Autodesk Fusion 360 part; units mm, degrees
sketch "Sketch1" plane through (0, 0, 0) normal (0, 0, 1) x (1, 0, 0)
  line L0 (50.6391, 82.0886) -> (110.6391, 82.0886)
  line L1 (110.6391, 82.0886) -> (110.6391, 22.0886)
  line L2 (110.6391, 22.0886) -> (50.6391, 22.0886)
  line L3 (50.6391, 22.0886) -> (50.6391, 82.0886)
  line L4 (55.6391, 77.0886) -> (105.6391, 77.0886)
  line L5 (105.6391, 77.0886) -> (105.6391, 27.0886)
  line L6 (105.6391, 27.0886) -> (55.6391, 27.0886)
  line L7 (55.6391, 27.0886) -> (55.6391, 77.0886)
  dimension "d1" = 60
  dimension "d2" = 60
  dimension "d5" = 50
  dimension "d6" = 50
extrude "Extrude1" add sketch "Sketch1" along normal blind 10 contours L4 L5 L6 L7
extrude "Extrude2" add sketch "Sketch1" along normal blind 60
sketch "Sketch2" plane through (0, 22.0886, 0) normal (0, -1, 0) x (1, 0, 0)
  line L0 (50.6391, 0) -> (110.6391, 0)
  line L1 (110.6391, 0) -> (110.6391, 60)
  line L2 (110.6391, 60) -> (50.6391, 60)
  line L3 (50.6391, 60) -> (50.6391, 0)
  line L4 (80.6391, 35) -> (75.6391, 35)
  line L5 (75.6391, 35) -> (85.6391, 35)
  line L6 (85.6391, 35) -> (85.6391, 25)
  line L7 (85.6391, 25) -> (75.6391, 25)
  line L8 (75.6391, 25) -> (75.6391, 35)
  dimension "d13" = 10
  dimension "d14" = 10
extrude "Extrude3" cut sketch "Sketch2" against normal blind 3.3 contours L4 L5 L6 L7 L8
Input: part model. Units: mm. Frame: model coordinates. A direction names the side the tool comes from. Give positions to 0.01 mm unless a question says otherwise; leave off trailing zeros. Order: outer loops, then holes, each group sorted by start corner. A loop starts at its lowest first (then second) coordinate and runs counter-clockwise, first axis right, second up. Notation, with made-up numbers: (-9, 25.25) - (2, 25.25) arc R16 cw to (2, 48.25) - close; hole circle Ø10 at (-1, -29.5). An arc over 180 degrees is marked (long way). Use a Markdown table: item, result.
(1) Section query A-A (x = 104.5). Output: boundary loops of the cut face in (y, z), then the cut area to 3 significant figures.
Computed values:
| item | result |
|---|---|
| outline | (22.09, 0) - (82.09, 0) - (82.09, 60) - (77.09, 60) - (77.09, 10) - (27.09, 10) - (27.09, 60) - (22.09, 60) - close |
| area | 1,100 mm2 |
(2) Draft query along Z for faces 1 (the flat face through (80, 52, 10)), 2 (the flat face through (80, 53, 0)), 3 (the flat face through (81, 24, 25)), 4 (the flat face through (55.639, 52, 35)). Return one class per face: released by +Z, released by -Z, zero draft, split by the parting line, or undercut.
Computed values:
| item | result |
|---|---|
| face 1 | released by +Z |
| face 2 | released by -Z |
| face 3 | undercut |
| face 4 | zero draft |
(3) Pin query (flat end, axial travel): pin 1 (4 mm diameter, centred on x = 78, y = 58.5, fed in from +Z). Return the tip coordinate at first contact, or that it passes through.
Computed values:
| item | result |
|---|---|
| pin 1 | stops at z = 10 |
(4) Access query for faces 5 (the flat face through (81, 27.089, 35)), 6 (the flat face through (75.639, 24, 30)), 7 (the flat face through (88, 22.089, 30)). Directions: +Z, -Z, +X, -X, +Y, -Y. A direction counts if a zero-diameter tool reaches every point of the face in a straight line with its end or side. Return the directions, or none.
Computed values:
| item | result |
|---|---|
| face 5 | +Z |
| face 6 | -Y |
| face 7 | +Z, -Z, +X, -X, -Y |
(5) Line query: line 1 (X direction, y = 33.5, z = 48.5); line 2 (Y direction, x = 91, z = 42); line 3 (Z direction, x = 77, y = 59). Output: solid intervals per line, ascending. Write a range as from..to.
Computed values:
| item | result |
|---|---|
| line 1 | x = 50.64..55.64, 105.64..110.64 |
| line 2 | y = 22.09..27.09, 77.09..82.09 |
| line 3 | z = 0..10 |
(6) Section query C-C (z = 36). Output: boundary loops of the cut face in (x, y), then the cut area to 3 significant figures.
Computed values:
| item | result |
|---|---|
| outline | (50.64, 22.09) - (110.64, 22.09) - (110.64, 82.09) - (50.64, 82.09) - close; hole (55.64, 27.09) - (105.64, 27.09) - (105.64, 77.09) - (55.64, 77.09) - close |
| area | 1,100 mm2 |
(7) Section query B-B (y = 44). Output: boundary loops of the cut face in (x, z).
Computed values:
| item | result |
|---|---|
| outline | (50.64, 0) - (110.64, 0) - (110.64, 60) - (105.64, 60) - (105.64, 10) - (55.64, 10) - (55.64, 60) - (50.64, 60) - close |
